```python
from build123d import *

# Parameters (mm, degrees)
EXTRUDE_DEPTH   = 3.3
SKETCH001_R     = 1.5
POCKET_DEPTH    = 3.301
SKETCH002_R     = 3
POCKET001_DEPTH = 5


with BuildPart() as part:
    # Sketch → Extrude (new body)
    with BuildSketch(Plane.XY):
        with BuildLine():
            ThreePointArc((3.5, 21.5), (0, 25), (-3.5, 21.5))
            Line((-3.5, 21.5), (-3.5, 19.691369))
            ThreePointArc((-3.5, 19.691369), (0, -20), (3.5, 19.691369))
            Line((3.5, 19.691369), (3.5, 21.5))
        make_face()
    extrude(amount=EXTRUDE_DEPTH)

    # Sketch001 (on Face6 of Extrude) → Pocket (cut, through all)
    with BuildSketch(Plane.XY.offset(3.3)):
        with Locations((0, 21.5)):
            Circle(SKETCH001_R)
    extrude(amount=-POCKET_DEPTH, mode=Mode.SUBTRACT)

    # Sketch002 (on Face6 of BaseFeature) → Pocket001 (cut)
    with BuildSketch(Plane.XY.offset(3.3)):
        with Locations((9, 9)):
            Circle(SKETCH002_R)
        with Locations((-9, 9)):
            Circle(SKETCH002_R)
        with BuildLine():
            ThreePointArc((-13, -7.483315), (0, -15), (13, -7.483315))
            Line((6.5, -7.483315), (13, -7.483315))
            Line((6.5, -10.483315), (6.5, -7.483315))
            Line((1.5, -10.483315), (6.5, -10.483315))
            Line((1.5, -7.483315), (1.5, -10.483315))
            Line((-1.5, -7.483315), (1.5, -7.483315))
            Line((-1.5, -10.483315), (-1.5, -7.483315))
            Line((-6.5, -10.483315), (-1.5, -10.483315))
            Line((-6.5, -7.483315), (-6.5, -10.483315))
            Line((-6.5, -7.483315), (-13, -7.483315))
        make_face()
    extrude(amount=-POCKET001_DEPTH, mode=Mode.SUBTRACT)


solid = part.part
```
Could you check a few things on this model? Use its own coordinates, in mm. A direction names the side the tool comes from. Coordinates: 2 decimals unless noted, no trailing zeros. Write each loop counter-clockwise with the first axis right and the second up, starting at its lowest first coordinate (ties: lowest second). Pieces come first, ordered by that corner, then holes. Notation, with made-up numbers: (89, 30.5) -> (114, 30.5) arc R23 cw to (114, 58.5) -> close; hole circle Ø10 at (3.25, 28.25). An arc over 180 degrees is marked (long way). One line per question, with ' | ' between items. Start each with the question number.
1. If we section it at C-C (y = 9.5): Please give me the cut outline in (x, z), and give its area (3 significant figures).
2. If we section it at B-B (x = 0): Please give me the cut outline in (y, z).
3. Will these pins go through, and if not, where does the flat tip stop? P1, Ø0.9, axis at y = -9.5, z = 1.5, coming from the -X side; P2, Ø0.9, axis at y = -9.5, z = 1.5, coming from the +X side; P3, Ø1, axis at x = -10.5, z = 1, coming from the -Y side; P4, Ø3.5, axis at x = -9, y = 9, coming from the +Z side.
4. Thinking about a two-plate mould opening in Y: for faces 1 (the face through (0, 3, 0)), 2 (the face through (4, -10.483, 2)), 3 (the face through (-0.83, -19.983, 1.627)), which applies, pulls with the +Y half, pulls with the -Y half, needs draft (parallel to the pull), parting line crosses it, or undercut?
5. If we section it at D-D (y = -9.5): Please give me the cut outline in (x, z).
6. For faces 4 (the face through (0, 3, 3.3)), 5 (the face through (-6.5, -9, 2)), 6 (the face through (0, 25, 2)), 7 (the face through (-3.5, 21, 2)), 8 (the face through (3.5, 21, 2)), which set-ups out of +Z, -Z, +X, -X, +Y, -Y let a thin tool reach every point of the face, with its end or its side?
7. Please list where these lines run through material, in increasing order: line 1 along Y through (x, z) = (11.5, 1.65); line 2 along Y through (x, z) = (-10, 1); line 3 along X through (y, z) = (-8, 1.45).
8. If we section it at A-A (z = 1.3): Please give me the cut outline in (x, y).
Return value:
1) outline: (-17.6, 0) -> (-11.96, 0) -> (-11.96, 3.3) -> (-17.6, 3.3) -> close; (-6.04, 0) -> (6.04, 0) -> (6.04, 3.3) -> (-6.04, 3.3) -> close; (11.96, 0) -> (17.6, 0) -> (17.6, 3.3) -> (11.96, 3.3) -> close | area: 77.1 mm²
2) outline: (-20, 0) -> (-15, 0) -> (-15, 3.3) -> (-20, 3.3) -> close; (-7.48, 0) -> (20, 0) -> (20, 3.3) -> (-7.48, 3.3) -> close; (23, 0) -> (25, 0) -> (25, 3.3) -> (23, 3.3) -> close
3) P1: stops at x = -17.84 | P2: stops at x = 17.84 | P3: stops at y = -17.32 | P4: passes through
4) face 1: needs draft | face 2: undercut | face 3: parting line crosses it
5) outline: (-17.6, 0) -> (-11.61, 0) -> (-11.61, 3.3) -> (-17.6, 3.3) -> close; (-6.5, 0) -> (-1.5, 0) -> (-1.5, 3.3) -> (-6.5, 3.3) -> close; (1.5, 0) -> (6.5, 0) -> (6.5, 3.3) -> (1.5, 3.3) -> close; (11.61, 0) -> (17.6, 0) -> (17.6, 3.3) -> (11.61, 3.3) -> close
6) face 4: +Z, +X, -X, +Y, -Y | face 5: +Z, -Z | face 6: +Z, -Z, +Y | face 7: +Z, -Z, -X, +Y | face 8: +Z, -Z, +X, +Y
7) line 1: y = -16.36 to -9.63, -7.48 to 7.34, 10.66 to 16.36 | line 2: y = -17.32 to -11.18, -7.48 to 6.17, 11.83 to 17.32 | line 3: x = -18.33 to -12.69, -6.5 to -1.5, 1.5 to 6.5, 12.69 to 18.33
8) outline: (-3.5, 19.69) arc R20 ccw (long way) to (3.5, 19.69) -> (3.5, 21.5) arc R3.5 ccw to (-3.5, 21.5) -> close; hole (-13, -7.48) arc R15 ccw to (13, -7.48) -> (6.5, -7.48) -> (6.5, -10.48) -> (1.5, -10.48) -> (1.5, -7.48) -> (-1.5, -7.48) -> (-1.5, -10.48) -> (-6.5, -10.48) -> (-6.5, -7.48) -> close; hole circle Ø6 at (-9, 9); hole circle Ø3 at (0, 21.5); hole circle Ø6 at (9, 9)
